```python
from build123d import *

# Parameters (mm, degrees)
SKETCH1_W               = 190
SKETCH1_H               = 85
BOSS_EXTRUDE1_DEPTH     = 6
SKETCH2_W               = 20
SKETCH2_H               = 9
BOSS_EXTRUDE2_DEPTH     = 38
SKETCH3_R               = 1.175
SKETCH3_W               = 12.35
SKETCH3_H               = 23
CUT_EXTRUDE1_DEPTH      = 30
MIRROR2_COPY_1_SKETCH_W = 20
MIRROR2_COPY_1_SKETCH_H = 9
MIRROR2_COPY_1_DEPTH    = 38
MIRROR2_COPY_2_SKETCH_R = 1.175
MIRROR2_COPY_2_SKETCH_W = 12.35
MIRROR2_COPY_2_SKETCH_H = 23
MIRROR2_COPY_2_DEPTH    = 30
SKETCH10_R              = 1.6
CUT_EXTRUDE2_DEPTH      = 6
SKETCH11_R              = 2.1
CUT_EXTRUDE3_DEPTH      = 10
SKETCH15_W              = 74
SKETCH15_H              = 25
CUT_EXTRUDE5_DEPTH      = 10
FILLET3_R               = 3
SKETCH16_R              = 2.1
CUT_EXTRUDE6_DEPTH      = 10
SKETCH13_R              = 1.175
CUT_EXTRUDE7_DEPTH      = 10


with BuildPart() as part:
    # Sketch1 → Boss-Extrude1 (new body)
    with BuildSketch(Plane(origin=(0, 0, 0), x_dir=(1, 0, 0), z_dir=(0, 1, 0))):
        Rectangle(SKETCH1_W, SKETCH1_H)
    extrude(amount=BOSS_EXTRUDE1_DEPTH)

    # Sketch2 → Boss-Extrude2 (add)
    with BuildSketch(Plane(origin=(0, 6, 0), x_dir=(1, 0, 0), z_dir=(0, 1, 0))):
        with Locations((70, -38)):
            Rectangle(SKETCH2_W, SKETCH2_H)
    boss_extrude2 = extrude(amount=BOSS_EXTRUDE2_DEPTH)

    # Sketch3 → Cut-Extrude1 (cut)
    with BuildSketch(Plane.XY.offset(42.5)):
        with Locations((70, 38.67)):
            Circle(SKETCH3_R)
        with Locations((70, 11.03)):
            Circle(SKETCH3_R)
        with Locations((70, 24.85)):
            Rectangle(SKETCH3_W, SKETCH3_H)
    cut_extrude1 = extrude(amount=-CUT_EXTRUDE1_DEPTH, mode=Mode.SUBTRACT)

    # Mirror1: Boss-Extrude2, Cut-Extrude1 across plane
    add(boss_extrude2.mirror(Plane.XY))
    add(cut_extrude1.mirror(Plane.XY), mode=Mode.SUBTRACT)

    # Mirror2: Boss-Extrude2, Cut-Extrude1 across plane
    add(boss_extrude2.mirror(Plane.ZY))
    add(cut_extrude1.mirror(Plane.ZY), mode=Mode.SUBTRACT)

    # Mirror2 copy 1 sketch → Mirror2 copy 1 (add)
    with BuildSketch(Plane(origin=(0, 6, 0), x_dir=(-1, 0, 0), z_dir=(0, 1, 0))):
        with Locations((70, -38)):
            Rectangle(MIRROR2_COPY_1_SKETCH_W, MIRROR2_COPY_1_SKETCH_H)
    extrude(amount=MIRROR2_COPY_1_DEPTH)

    # Mirror2 copy 2 sketch → Mirror2 copy 2 (cut)
    with BuildSketch(Plane(origin=(0, 0, -42.5), x_dir=(-1, 0, 0), z_dir=(0, 0, -1))):
        with Locations((70, 38.67)):
            Circle(MIRROR2_COPY_2_SKETCH_R)
        with Locations((70, 11.03)):
            Circle(MIRROR2_COPY_2_SKETCH_R)
        with Locations((70, 24.85)):
            Rectangle(MIRROR2_COPY_2_SKETCH_W, MIRROR2_COPY_2_SKETCH_H)
    extrude(amount=-MIRROR2_COPY_2_DEPTH, mode=Mode.SUBTRACT)

    # Sketch10 → Cut-Extrude2 (cut)
    with BuildSketch(Plane(origin=(0, 6, 0), x_dir=(1, 0, 0), z_dir=(0, 1, 0))):
        with Locations(Location((31.7, 24.1, 0), (0, 0, 270))):
            Circle(SKETCH10_R)
        with Locations(Location((82.5, 8.9, 0), (0, 0, 270))):
            Circle(SKETCH10_R)
        with Locations(Location((82.5, -19, 0), (0, 0, 270))):
            Circle(SKETCH10_R)
        with Locations(Location((30.4, -24.1, 0), (0, 0, 270))):
            Circle(SKETCH10_R)
    extrude(amount=-CUT_EXTRUDE2_DEPTH, mode=Mode.SUBTRACT)

    # Sketch11 → Cut-Extrude3 (cut)
    with BuildSketch(Plane(origin=(0, 6, 0), x_dir=(1, 0, 0), z_dir=(0, 1, 0))):
        with Locations(Location((88, 34, 0), (0, 0, 270))):
            Circle(SKETCH11_R)
        with Locations(Location((88, -34, 0), (0, 0, 270))):
            Circle(SKETCH11_R)
        with Locations(Location((-88, 34, 0), (0, 0, 270))):
            Circle(SKETCH11_R)
        with Locations(Location((-88, -34, 0), (0, 0, 270))):
            Circle(SKETCH11_R)
    extrude(amount=-CUT_EXTRUDE3_DEPTH, mode=Mode.SUBTRACT)

    # Sketch15 → Cut-Extrude5 (cut)
    with BuildSketch(Plane(origin=(0, 6, 0), x_dir=(1, 0, 0), z_dir=(0, 1, 0))):
        with Locations((-13, 30)):
            Rectangle(SKETCH15_W, SKETCH15_H)
        with Locations((-13, -30)):
            Rectangle(SKETCH15_W, SKETCH15_H)
    extrude(amount=-CUT_EXTRUDE5_DEPTH, mode=Mode.SUBTRACT)

    # Fillet3
    fillet3_edges = [part.edges().sort_by_distance(p)[0] for p in [
        (-50, 3, -17.5),
        (24, 3, -17.5),
        (-50, 3, 17.5),
        (24, 3, 17.5),
    ]]
    fillet(fillet3_edges, radius=FILLET3_R)

    # Sketch16 → Cut-Extrude6 (cut)
    with BuildSketch(Plane(origin=(0, 6, 0), x_dir=(1, 0, 0), z_dir=(0, 1, 0))):
        with Locations(Location((91, 6, 0), (0, 0, 270))):
            Circle(SKETCH16_R)
        with Locations(Location((91, -6, 0), (0, 0, 270))):
            Circle(SKETCH16_R)
        with Locations(Location((-91, 6, 0), (0, 0, 270))):
            Circle(SKETCH16_R)
        with Locations(Location((-91, -6, 0), (0, 0, 270))):
            Circle(SKETCH16_R)
    extrude(amount=-CUT_EXTRUDE6_DEPTH, mode=Mode.SUBTRACT)

    # Sketch13 → Cut-Extrude7 (cut)
    with BuildSketch(Plane(origin=(0, 6, 0), x_dir=(1, 0, 0), z_dir=(0, 1, 0))):
        with Locations(Location((-4.45, 7.775, 0), (0, 0, 270))):
            Circle(SKETCH13_R)
        with Locations(Location((-4.45, -7.775, 0), (0, 0, 270))):
            Circle(SKETCH13_R)
        with Locations(Location((-80, 7.775, 0), (0, 0, 270))):
            Circle(SKETCH13_R)
        with Locations(Location((-80, -7.775, 0), (0, 0, 270))):
            Circle(SKETCH13_R)
    extrude(amount=-CUT_EXTRUDE7_DEPTH, mode=Mode.SUBTRACT)


solid = part.part
```
Work out the finished part from the listing and answer in its coordinate system (mm). A direction names the side the tool comes from. Give positions to 0.01 mm unless a question says otherwise; leave off trailing zeros. Order: outer loops, then holes, each group sorted by start corner. A loop starts at its lowest first (then second) coordinate and runs counter-clockwise, first axis right, second up.
1. For faces 5 (the flat face through (-63, 25, 33.5)), 6 (the flat face through (-13, 3, 17.5)), 7 (the flat face through (65, 10, -42.5)), 8 (the flat face through (76.175, 25, 38)), determine the directions among +Z, -Z, +X, -X, +Y, -Y from which every point of the face is accessible in a straight line to the end or side of a thin tool.
Result sheet:
face 5: +X, -X, +Y
face 6: +Z, +Y, -Y
face 7: -Z, +X, -X, +Y, -Y
face 8: +Z, -Z
2. The mould has two halves that part along X. Classify faces 1 (the flat face through (80, 25, 38)), 2 (the cylindrical face through (-92.278, 3.042, 4.334)), 3 (the cylindrical face through (89.722, 3.042, 4.334)), 4 (the flat face through (-70, 44, 38)): released by +X, released by -X, zero draft, split by the parting line, or undercut.
Result sheet:
face 1: released by +X
face 2: undercut
face 3: undercut
face 4: zero draft
3. Straight lines are drawn through the part: L1, parallel to X at y = 29.5, z = -34 (3 decimals); L2, parallel to X at y = 3, z = -34; L3, parallel to Y at x = 70, z = -38 (3 decimals). For each, find the intervals that lie inside material, in ascending order.
Result sheet:
L1: x = -80 to -76.175, -63.825 to -60, 60 to 63.825, 76.175 to 80
L2: x = -95 to -90.1, -85.9 to -50, 24 to 85.9, 90.1 to 95
L3: y = 0 to 9.855, 12.205 to 13.35, 36.35 to 37.495, 39.845 to 44
4. Section A-A, the plane z = 14 is taken. Determine the outline of the cut face in (x, y).
Result sheet:
outline: (-95, 0) - (95, 0) - (95, 6) - (-95, 6) - close
5. Section B-B, the plane x = -16.5 is taken. Determine the outline of the cut face in (y, z).
Result sheet:
outline: (0, -17.5) - (6, -17.5) - (6, 17.5) - (0, 17.5) - close
6. Each of these flat-tipped pins is pushed along its axis until it touches: P1, Ø10, axis at y = 22, z = 38, coming from the -X side; P2, Ø3.5, axis at x = -91, z = 6, coming from the -Y side; P3, Ø2.5, axis at x = -80, z = 7.775, coming from the -Y side; P4, Ø5, axis at x = 88, z = -34, coming from the +Y side. Where does it stop, or does it pass through?
Result sheet:
P1: stops at x = -80
P2: passes through
P3: stops at y = 0
P4: stops at y = 6
